from build123d import *

# Parameters (mm, degrees)
SKETCH1_R            = 9.35
SKETCH1_R_2          = 7.95
BOSS_EXTRUDE1_DEPTH  = 31.6
SKETCH2_R            = 3.05
SKETCH2_R_2          = 1.15
BOSS_EXTRUDE2_DEPTH  = 45
BOSS_EXTRUDE3_DEPTH  = 18.45
SKETCH5_W            = 7.65
SKETCH5_H            = 14.65
CUT_EXTRUDE1_DEPTH   = 15
SKETCH6_R            = 7.95
SKETCH6_R_2          = 3.05
BOSS_EXTRUDE4_DEPTH  = 0.2
CUT_EXTRUDE4_DEPTH   = 0.2
BOSS_EXTRUDE5_DEPTH  = 7.45
BOSS_EXTRUDE6_DEPTH  = 1.7
BOSS_EXTRUDE7_START  = -1.7
SKETCH10_R           = 2.5
SKETCH10_R_2         = 1
BOSS_EXTRUDE7_DEPTH  = 7.7
BOSS_EXTRUDE8_DEPTH  = 1.7
BOSS_EXTRUDE9_DEPTH  = 5
SKETCH13_R           = 9.35
SKETCH13_R_2         = 7.95
BOSS_EXTRUDE12_DEPTH = 2
BOSS_EXTRUDE13_DEPTH = 1.7
CUT_EXTRUDE5_DEPTH   = 0.9
BOSS_EXTRUDE14_DEPTH = 0.9


with BuildPart() as part:
    # Sketch1 → Boss-Extrude1 (new body)
    with BuildSketch(Plane(origin=(0, 0, 0), x_dir=(1, 0, 0), z_dir=(0, 1, 0))):
        Circle(SKETCH1_R)
        Circle(SKETCH1_R_2, mode=Mode.SUBTRACT)
    extrude(amount=BOSS_EXTRUDE1_DEPTH)

    # Sketch4 → Boss-Extrude3 (add)
    with BuildSketch(Plane(origin=(0, 7.3, 0), x_dir=(1, 0, 0), z_dir=(0, 1, 0))):
        with BuildLine():
            Line((19.392352467, 5.725), (7.392352467, 5.725))
            ThreePointArc((7.392352467, 5.725), (9.266531417, -1.24655345), (5.616660485, -7.475))
            Line((5.616660485, -7.475), (10.416660485, -7.475))
            ThreePointArc((10.416660485, -7.475), (11.654097352, -6.962436867), (12.166660485, -5.725))
            Line((12.166660485, -5.725), (19.392352467, -5.725))
            Line((19.392352467, -5.725), (19.392352467, 5.725))
        make_face()
    extrude(amount=BOSS_EXTRUDE3_DEPTH)

    # Sketch5 → Cut-Extrude1 (cut)
    with BuildSketch(Plane(origin=(19.392352467, 0, 0), x_dir=(0, 0, -1), z_dir=(1, 0, 0))):
        with Locations((0, 16.525)):
            Rectangle(SKETCH5_W, SKETCH5_H)
    extrude(amount=-CUT_EXTRUDE1_DEPTH, mode=Mode.SUBTRACT)



with BuildPart() as body_2:
    # Sketch2 → Boss-Extrude2 (new body)
    with BuildSketch(Plane(origin=(0, -3.3, 0), x_dir=(1, 0, 0), z_dir=(0, 1, 0))):
        Circle(SKETCH2_R)
        Circle(SKETCH2_R_2, mode=Mode.SUBTRACT)
    extrude(amount=BOSS_EXTRUDE2_DEPTH)


with BuildPart() as part_1:
    add(part.part)

    add(body_2.part)  # Boss-Extrude4 merges body 2
    # Sketch6 → Boss-Extrude4 (add)
    with BuildSketch(Plane(origin=(0, 16, 0), x_dir=(1, 0, 0), z_dir=(0, 1, 0))):
        Circle(SKETCH6_R)
        Circle(SKETCH6_R_2, mode=Mode.SUBTRACT)
    extrude(amount=BOSS_EXTRUDE4_DEPTH)

    # Sketch7 → Cut-Extrude4 (cut)
    with BuildSketch(Plane(origin=(0, 16, 0), x_dir=(1, 0, 0), z_dir=(0, 1, 0))):
        with BuildLine():
            Line((6.969352552, 3.825), (1.069352552, 3.825))
            Line((1.069352552, 3.825), (1.069352552, 2.856393726))
            ThreePointArc((1.069352552, 2.856393726), (3.05, 0), (1.069352552, -2.856393726))
            Line((1.069352552, -2.856393726), (1.069352552, -3.825))
            Line((1.069352552, -3.825), (6.969352552, -3.825))
            ThreePointArc((6.969352552, -3.825), (7.95, 0), (6.969352552, 3.825))
        make_face()
    extrude(amount=CUT_EXTRUDE4_DEPTH, mode=Mode.SUBTRACT)

    # Sketch8 → Boss-Extrude5 (add)
    with BuildSketch(Plane(origin=(0, 20.6, 0), x_dir=(1, 0, 0), z_dir=(0, 1, 0))):
        with BuildLine():
            Line((-4.4, -8.25), (-7.403469592, -8.25))
            ThreePointArc((-7.403469592, -8.25), (-7.894744058, -8.066700449), (-8.145884154, -7.606398397))
            ThreePointArc((-8.145884154, -7.606398397), (-8.681216078, -6.028326508), (-9.750221455, -4.75))
            Line((-9.750221455, -4.75), (-8.451183349, -4))
            ThreePointArc((-8.451183349, -4), (-6.767854414, -6.451251555), (-4.4, -8.25))
        make_face()
    extrude(amount=BOSS_EXTRUDE5_DEPTH)

    # Sketch12 → Boss-Extrude9 (add)
    with BuildSketch(Plane.XZ.offset(-20.6)):
        with BuildLine():
            Line((-4.4, 8.25), (-7.403469592, 8.25))
            ThreePointArc((-7.403469592, 8.25), (-7.894744058, 8.066700449), (-8.145884154, 7.606398397))
            ThreePointArc((-8.145884154, 7.606398397), (-8.681216078, 6.028326508), (-9.750221455, 4.75))
            Line((-9.750221455, 4.75), (-8.451183349, 4))
            ThreePointArc((-8.451183349, 4), (-6.767854414, 6.451251555), (-4.4, 8.25))
        make_face()
    extrude(amount=BOSS_EXTRUDE9_DEPTH)



with BuildPart() as body_2_2:
    # Sketch9 → Boss-Extrude6 (new body)
    with BuildSketch(Plane(origin=(0, 31.6, 0), x_dir=(1, 0, 0), z_dir=(0, 1, 0))):
        with BuildLine():
            Line((-8.328265125, 4.25), (-10.822291045, 5.522727273))
            Line((-10.822291045, 5.522727273), (-17.029180659, -6.640242682))
            Line((-17.029180659, -6.640242682), (-14.089792968, -8.140242682))
            ThreePointArc((-14.089792968, -8.140242682), (-11.800883152, -8.321818546), (-10.053985976, -6.831708418))
            Line((-10.053985976, -6.831708418), (-8.526111367, -3.837697872))
            ThreePointArc((-8.526111367, -3.837697872), (-9.347203644, 0.228657047), (-8.328265125, 4.25))
        make_face()
    extrude(amount=-BOSS_EXTRUDE6_DEPTH)

    # Sketch10 → Boss-Extrude7 (add)
    with BuildSketch(Plane(origin=(0, 31.6, 0), x_dir=(1, 0, 0), z_dir=(0, 1, 0)).offset(BOSS_EXTRUDE7_START)):
        with Locations((-14.802371802, -7.776606319)):
            Circle(SKETCH10_R)
        with Locations((-14.802371802, -7.776606319)):
            Circle(SKETCH10_R_2, mode=Mode.SUBTRACT)
    extrude(amount=BOSS_EXTRUDE7_DEPTH)

    # Sketch11 → Boss-Extrude8 (add)
    with BuildSketch(Plane(origin=(0, 31.6, 0), x_dir=(1, 0, 0), z_dir=(0, 1, 0))):
        with BuildLine():
            Line((-15.693095345, -7.322060864), (-14.089792968, -8.140242682))
            ThreePointArc((-14.089792968, -8.140242682), (-13.999922503, -8.184231187), (-13.908635087, -8.225198209))
            ThreePointArc((-13.908635087, -8.225198209), (-15.253942988, -8.668841413), (-15.693095345, -7.322060864))
        make_face()
    extrude(amount=-BOSS_EXTRUDE8_DEPTH)


with BuildPart() as part_2:
    add(part_1.part)

    add(body_2_2.part)  # Boss-Extrude12 merges body 2 2
    # Sketch13 → Boss-Extrude12 (add)
    with BuildSketch(Plane(origin=(0, 31.6, 0), x_dir=(1, 0, 0), z_dir=(0, 1, 0))):
        Circle(SKETCH13_R)
        Circle(SKETCH13_R_2, mode=Mode.SUBTRACT)
    extrude(amount=BOSS_EXTRUDE12_DEPTH)

    # Sketch14 → Boss-Extrude13 (add)
    with BuildSketch(Plane(origin=(0, 31.6, 0), x_dir=(1, 0, 0), z_dir=(0, 1, 0))):
        with BuildLine():
            Line((-10.053985976, -6.831708418), (-8.526111367, -3.837697872))
            ThreePointArc((-8.526111367, -3.837697872), (-9.347203644, 0.228657047), (-8.328265125, 4.25))
            Line((-8.328265125, 4.25), (-10.822291045, 5.522727273))
            Line((-10.822291045, 5.522727273), (-17.029180659, -6.640242682))
            ThreePointArc((-17.029180659, -6.640242682), (-15.711611281, -10.105400764), (-12.394688357, -8.449703956))
            ThreePointArc((-12.394688357, -8.449703956), (-11.020302269, -7.935876946), (-10.053985976, -6.831708418))
        make_face()
    extrude(amount=-BOSS_EXTRUDE13_DEPTH)

    # Sketch15 → Cut-Extrude5 (cut)
    with BuildSketch(Plane.XZ.offset(-29.9)):
        with BuildLine():
            Line((-17.029180659, 6.640242682), (-10.822291045, -5.522727273))
            Line((-10.822291045, -5.522727273), (-8.328265125, -4.25))
            ThreePointArc((-8.328265125, -4.25), (-9.347203644, -0.228657047), (-8.526111367, 3.837697872))
            Line((-8.526111367, 3.837697872), (-10.053985976, 6.831708418))
            ThreePointArc((-10.053985976, 6.831708418), (-11.020302269, 7.935876946), (-12.394688357, 8.449703956))
            ThreePointArc((-12.394688357, 8.449703956), (-15.711611281, 10.105400764), (-17.029180659, 6.640242682))
        make_face()
    extrude(amount=-CUT_EXTRUDE5_DEPTH, mode=Mode.SUBTRACT)

    # Sketch17 → Boss-Extrude14 (add)
    with BuildSketch(Plane(origin=(0, 31.6, 0), x_dir=(1, 0, 0), z_dir=(0, 1, 0))):
        with BuildLine():
            Line((-10.053985976, -6.831708418), (-8.526111367, -3.837697872))
            ThreePointArc((-8.526111367, -3.837697872), (-9.347203644, 0.228657047), (-8.328265125, 4.25))
            Line((-8.328265125, 4.25), (-10.822291045, 5.522727273))
            Line((-10.822291045, 5.522727273), (-17.029180659, -6.640242682))
            ThreePointArc((-17.029180659, -6.640242682), (-15.711611281, -10.105400764), (-12.394688357, -8.449703956))
            ThreePointArc((-12.394688357, -8.449703956), (-11.020302269, -7.935876946), (-10.053985976, -6.831708418))
        make_face()
    extrude(amount=BOSS_EXTRUDE14_DEPTH)


solid = part_2.part
Could you check a few things on this model? Use its own coordinates, in mm. A direction names the side the tool comes from. Round coordinates to 2 decimals unless told otherwise and drop trailing zeros. Order: outer loops, then holes, each group sorted by start corner. A loop starts at its lowest first (then second) coordinate and runs counter-clockwise, first axis right, second up.
Q1. Please list where these lines run through material, in increasing order: probe 1 along X at (y, z) = (11.25, 0); probe 2 along Z at (x, y) = (0, 21.5).
Geometry says:
probe 1: x = -9.35 to -7.95, -3.05 to -1.15, 1.15 to 3.05
probe 2: z = -9.35 to -7.95, -3.05 to -1.15, 1.15 to 3.05, 7.95 to 9.35
Q2. Which directions (+Z, -Z, +X, -X, +Y, -Y) give clear straight access to the entire face, cutting with the end or side of a thin tool? Please do faces 1 (the face through (-8.67, 21.91, 6.05)), 2 (the face through (-4, 16, 0)), 3 (the face through (-9.301, 31.638, 5.356)), 4 (the face through (12, 16, 3.825)), 5 (the face through (-15.34, 34.15, 10.22)).
Geometry says:
face 1: +Z, -X, -Y
face 2: -Y
face 3: +Z, +Y
face 4: +X
face 5: +Y
Q3. Imagine slicing it at D-D, the plane z = 0. State how many separate pieces and enclosed holes the cut face has, then the cut area to 3 significant figures.
Geometry says:
separate pieces: 4
enclosed holes: 0
area: 291 mm2
Q4. I'm going to push flat-ended pins straight in: P1, Ø1.5, axis at y = 33.5, z = 4.5, coming from the +X side; P2, Ø2, axis at x = -14.5, z = 7.5, coming from the +Y side; P3, Ø12, axis at x = 14.5, y = 5.5, coming from the +Z side (3 decimals). Where does each tip first touch, or does it pass through?
Geometry says:
P1: stops at x = 8.57
P2: stops at y = 37.6
P3: stops at z = 7.475
Q5. Imagine slicing it at B-B, the plane x = 14. List the corners of the cut face in (y, z) for me (3 decimals).
Geometry says:
outline: (7.3, -5.725) - (25.75, -5.725) - (25.75, 5.725) - (7.3, 5.725) - close; hole (9.2, -3.825) - (23.85, -3.825) - (23.85, 3.825) - (9.2, 3.825) - close
Q6. Thinking about a two-plate mould opening in Z: for faces 6 (the face through (-7.5, 15.6, 6.4)), 7 (the face through (-0.91, 18.88, 0.7)), 8 (the face through (13, 9.2, 0)), 9 (the face through (8, 16, 7.475)), which applies, released by +Z, released by -Z, zero draft, split by the parting line, or undercut?
Geometry says:
face 6: zero draft
face 7: undercut
face 8: undercut
face 9: released by +Z
Q7. Imagine slicing it at A-A, the plane y = 6.5. List the corners of the cut face in (x, z) for me, then the cut area to 3 significant figures.
Geometry says:
outline: circle Ø18.7 at (0, 0); circle Ø6.1 at (0, 0); hole circle Ø15.9 at (0, 0); hole circle Ø2.3 at (0, 0)
area: 101 mm2
Q8. Imagine slicing it at C-C, the plane x = 0. List the corners of the cut face in (y, z) for me, then the cut area to 3 significant figures.
Geometry says:
outline: (-3.3, -3.05) - (16, -3.05) - (16, -7.95) - (0, -7.95) - (0, -9.35) - (33.6, -9.35) - (33.6, -7.95) - (16.2, -7.95) - (16.2, -3.05) - (41.7, -3.05) - (41.7, -1.15) - (-3.3, -1.15) - close; (-3.3, 1.15) - (41.7, 1.15) - (41.7, 3.05) - (16.2, 3.05) - (16.2, 7.95) - (33.6, 7.95) - (33.6, 9.35) - (0, 9.35) - (0, 7.95) - (16, 7.95) - (16, 3.05) - (-3.3, 3.05) - close
area: 267 mm2
